```python
from build123d import *

# Parameters (mm, degrees)
SALIENTE_EXTRUIR1_DEPTH = 40
CORTAR_EXTRUIR4_DEPTH   = 36
SALIENTE_EXTRUIR2_DEPTH = 8.5
SALIENTE_EXTRUIR3_DEPTH = 40
CROQUIS5_R              = 2.15
CORTAR_EXTRUIR5_DEPTH   = 12
CORTAR_EXTRUIR7_DEPTH   = 30
CORTAR_EXTRUIR8_DEPTH   = 30
CROQUIS11_R             = 2.165
CORTAR_EXTRUIR9_DEPTH   = 30
CROQUIS12_R             = 2.15
CORTAR_EXTRUIR10_DEPTH  = 30


with BuildPart() as part:
    # Croquis2 → Saliente-Extruir1 (new body)
    with BuildSketch(Plane(origin=(0, 0, 0), x_dir=(1, 0, 0), z_dir=(0, 1, 0))):
        Polygon((0, 0), (48, 0), (48, 48), (30, 48), (30, 18), (0, 18), align=None)
    extrude(amount=SALIENTE_EXTRUIR1_DEPTH)

    # Croquis3 → Cortar-Extruir4 (cut)
    with BuildSketch(Plane(origin=(0, 40, 0), x_dir=(1, 0, 0), z_dir=(0, 1, 0))):
        Polygon((48, 14.142135624), (39.868272016, 22.273863607), (47.646446609, 30.0520382), (45.171572875, 32.526911935), (37.393398282, 24.748737342), (23.251262658, 10.606601718), (15.473088065, 2.828427125), (17.9479618, 0.353553391), (25.726136393, 8.131727984), (33.857864376, 0), (41.815185719, -7.957321343), (55.957321343, 6.184814281), align=None)
    extrude(amount=-CORTAR_EXTRUIR4_DEPTH, mode=Mode.SUBTRACT)

    # Croquis4 → Saliente-Extruir2 (add)
    with BuildSketch(Plane(origin=(0, 4, 0), x_dir=(1, 0, 0), z_dir=(0, 1, 0))):
        Polygon((39.868272016, 22.273863607), (37.393398282, 24.748737342), (45.171572875, 32.526911935), (47.646446609, 30.0520382), align=None)
        Polygon((15.473088065, 2.828427125), (17.9479618, 0.353553391), (25.726136393, 8.131727984), (23.251262658, 10.606601718), align=None)
    extrude(amount=SALIENTE_EXTRUIR2_DEPTH)

    # Croquis6 → Saliente-Extruir3 (add)
    with BuildSketch(Plane(origin=(0, 0, 0), x_dir=(1, 0, 0), z_dir=(0, 1, 0))):
        Polygon((30, 25.070901105), (22.929098895, 18), (30, 18), align=None)
    extrude(amount=SALIENTE_EXTRUIR3_DEPTH)

    # Croquis5 → Cortar-Extruir5 (cut)
    with BuildSketch(Plane(origin=(6.32233047, 0, 6.32233047), x_dir=(0.7071067811865472, 0, -0.7071067811865479), z_dir=(0.7071067811865479, 0, 0.7071067811865472))):
        with Locations((33.941125497, 8.5)):
            Circle(CROQUIS5_R)
    extrude(amount=-CORTAR_EXTRUIR5_DEPTH, mode=Mode.SUBTRACT)

    # Croquis9 → Cortar-Extruir7 (cut)
    with BuildSketch(Plane(origin=(0, 0, -18), x_dir=(-1, 0, 0), z_dir=(0, 0, -1))):
        Polygon((-22.929098895, 40), (-9, 5), (0, 5), (0, 40), align=None)
    extrude(amount=-CORTAR_EXTRUIR7_DEPTH, mode=Mode.SUBTRACT)

    # Croquis10 → Cortar-Extruir8 (cut)
    with BuildSketch(Plane.ZY.offset(-30)):
        Polygon((-25.070901105, 40), (-39, 5), (-48, 5), (-48, 40), align=None)
    extrude(amount=-CORTAR_EXTRUIR8_DEPTH, mode=Mode.SUBTRACT)

    # Croquis11 → Cortar-Extruir9 (cut)
    with BuildSketch(Plane(origin=(0, 5, 0), x_dir=(1, 0, 0), z_dir=(0, 1, 0))):
        with Locations(Location((39, 43.5, 0), (0, 0, 270))):
            Circle(CROQUIS11_R)
    extrude(amount=-CORTAR_EXTRUIR9_DEPTH, mode=Mode.SUBTRACT)

    # Croquis12 → Cortar-Extruir10 (cut)
    with BuildSketch(Plane(origin=(0, 5, 0), x_dir=(1, 0, 0), z_dir=(0, 1, 0))):
        with Locations(Location((4.5, 9, 0), (0, 0, 270))):
            Circle(CROQUIS12_R)
    extrude(amount=-CORTAR_EXTRUIR10_DEPTH, mode=Mode.SUBTRACT)


solid = part.part
```
The model under review builds one solid part; all positions refer to its coordinate system, in mm. A direction names the side the tool comes from. Round coordinates to 2 decimals unless told otherwise and drop trailing zeros. Loops run counter-clockwise (first coordinate to the right, second up) from the corner with the lowest first, then second, coordinate; pieces in that order, holes last. Notation, with made-up numbers: (51, -4) - (67, -4) arc R18 cw to (67, 12) - close; hole circle Ø3 at (-19, 22.25). An arc over 180 degrees is marked (long way). Write each question's results on one line, items separated by ' | '. Start each with the question number.
Q1. Tool access review of faces 1 (the flat face through (37, 5, -42)), 2 (the flat face through (21, 12.5, -6)), 3 (the flat face through (6, 5, -11)): name each direction out of +Z, -Z, +X, -X, +Y, -Y from which nothing blocks a thin tool from reaching the whole face with its end or side.
Q2. Take a section at A-A on x = 4.5. Give the boundary of the cut face in (y, z), plus the area to 3 significant figures.
Q3. Take a section at C-C on y = 32. Give the boundary of the cut face in (x, z), plus the area to 3 significant figures.
Q4. Take a section at B-B on z = -43.5. Give the boundary of the cut face in (x, y) (3 decimals), plus the area to 4 significant figures.
Q5. Take a section at D-D on x = 22. Give the boundary of the cut face in (y, z).
Q6. Draft analysis for pull direction X (two halves, no side actions). For faces 4 (the flat face through (26.51, 19.72, -21.58)), 5 (the flat face through (46.4, 18.4, -31.3)), 6 (the flat face through (27, 40, -3)), state which applies: pulls with the +X half, pulls with the -X half, needs draft (parallel to the pull), parting line crosses it, or undercut.
Q7. Insertion check: P1, Ø2.5, axis at x = 5.5, z = -8.5, coming from the +Y side; P2, Ø18.5, axis at y = 14.5, z = -33.5, coming from the -X side. Each pin has a flat end and moves straight along its axis. Give the tip position at first contact, or say it passes through.
Q8. Wall thickness on line 1 along X through (y, z) = (2, -9); line 2 along X through (y, z) = (3.5, -43.5) (3 decimals); line 3 along X through (y, z) = (4.5, -37.5): over which ranges is each line inside the solid? List them lowest first. Write a range as [from, to].
Data:
1) face 1: -Z, +X, -X, +Y | face 2: +Y | face 3: +Z, -Z, -X, +Y
2) outline: (0, -18) - (5, -18) - (5, -11.15) - (0, -11.15) - close; (0, -6.85) - (5, -6.85) - (5, 0) - (0, 0) - close | area: 68.5 mm²
3) outline: (19.75, -18) - (22.93, -18) - (30, -25.07) - (30, -28.25) - (40.9, -28.25) - (19.75, -7.1) - close; (19.75, -2.15) - (25.73, -8.13) - (33.86, 0) - (19.75, 0) - close; (39.87, -22.27) - (45.85, -28.25) - (48, -28.25) - (48, -14.14) - close | area: 271 mm²
4) outline: (30, 0) - (36.835, 0) - (36.835, 5) - (30, 5) - close; (41.165, 0) - (48, 0) - (48, 5) - (41.165, 5) - close | area: 68.35 mm²
5) outline: (0, -18) - (37.67, -18) - (37.67, -9.36) - (12.5, -9.36) - (12.5, -4.41) - (37.67, -4.41) - (37.67, 0) - (0, 0) - close
6) face 4: pulls with the -X half | face 5: undercut | face 6: needs draft
7) P1: stops at y = 5 | P2: stops at x = 29.18
8) line 1: x = [0, 2.35], [6.65, 48] | line 2: x = [30, 36.835], [41.165, 48] | line 3: x = [30, 48]
